Geometry: final body of the model. Coordinates: model frame, mm. A direction names the side the tool comes from. Round coordinates to 2 decimals unless told otherwise and drop trailing zeros. Loops run counter-clockwise (first coordinate to the right, second up) from the corner with the lowest first, then second, coordinate; pieces in that order, holes last. Notation, with made-up numbers: M 20,40.25 L 55,40.25 A25 cw 55,56.25 Z; hole C -37,5 d11. An arc over 180 degrees is marked long. Answer as a JSON object with one key per item and string values.
from build123d import *

# Parameters (mm, degrees)
F1_DEPTH = 1
F2_DEPTH = 11
F3_DEPTH = 10


with BuildPart() as f1:
    # F0 (on Top) → F1 (new body)
    with BuildSketch(Plane.XY):
        with BuildLine():
            ThreePointArc((12.3109959605, -2.4885695612), (12.4975939537, -1.250498048), (12.56, 0))
            ThreePointArc((12.56, 0), (12.499849565, 1.227746249), (12.3199743866, 2.4437330282))
            ThreePointArc((12.3199743866, 2.4437330282), (8.8241351782, 8.9380220607), (2.2855528975, 12.3502974844))
            ThreePointArc((2.2855528975, 12.3502974844), (0.0100228873, 12.5599960009), (-2.2658389037, 12.3539294988))
            ThreePointArc((-2.2658389037, 12.3539294988), (-8.8620220769, 8.9004586797), (-12.3440076572, 2.3192832854))
            ThreePointArc((-12.3440076572, 2.3192832854), (-12.559977123, 0.023972266), (-12.3527709674, -2.2721464362))
            ThreePointArc((-12.3527709674, -2.2721464362), (-8.8868925427, -8.8756262277), (-2.2878147001, -12.3498786997))
            ThreePointArc((-2.2878147001, -12.3498786997), (0.0002376292, -12.5599999978), (2.2882820061, -12.3497921222))
            ThreePointArc((2.2882820061, -12.3497921222), (8.8088397015, -8.9530968449), (12.3109959605, -2.4885695612))
        make_face()
        with BuildLine():
            ThreePointArc((12.3199743866, 2.4437330282), (12.499849565, 1.227746249), (12.56, 0))
            ThreePointArc((12.56, 0), (12.4975939537, -1.250498048), (12.3109959605, -2.4885695612))
            Line((12.3109959605, -2.4885695612), (13.1075011071, -2.5855424186))
            Line((13.1075011071, -2.5855424186), (14.1026028651, -2.7066940036))
            ThreePointArc((14.1026028651, -2.7066940036), (14.2955058872, -1.3594526209), (14.36, 0))
            ThreePointArc((14.36, 0), (14.2978344087, 1.334740133), (14.1118758743, 2.657923872))
            Line((14.1118758743, 2.657923872), (13.1166017889, 2.5389560617))
            Line((13.1166017889, 2.5389560617), (12.3199743866, 2.4437330282))
        make_face()
        with BuildLine():
            ThreePointArc((2.2855528975, 12.3502974844), (8.8241351782, 8.9380220607), (12.3199743866, 2.4437330282))
            Line((12.3199743866, 2.4437330282), (13.1166017889, 2.5389560617))
            Line((13.1166017889, 2.5389560617), (14.1118758743, 2.657923872))
            ThreePointArc((14.1118758743, 2.657923872), (10.136505033, 10.1715714477), (2.6091735777, 14.1209706905))
            Line((2.6091735777, 14.1209706905), (2.4293843449, 13.1372635399))
            Line((2.4293843449, 13.1372635399), (2.2855528975, 12.3502974844))
        make_face()
        with BuildLine():
            Line((13.1075011071, -2.5855424186), (12.3109959605, -2.4885695612))
            ThreePointArc((12.3109959605, -2.4885695612), (8.8088397015, -8.9530968449), (2.2882820061, -12.3497921222))
            Line((2.2882820061, -12.3497921222), (2.4340324524, -13.1364030853))
            Line((2.4340324524, -13.1364030853), (2.6162205102, -14.1196667893))
            ThreePointArc((2.6162205102, -14.1196667893), (10.1214500303, -10.1865523748), (14.1026028651, -2.7066940036))
            Line((14.1026028651, -2.7066940036), (13.1075011071, -2.5855424186))
        make_face()
        with BuildLine():
            ThreePointArc((-2.2658389037, 12.3539294988), (0.0100228873, 12.5599960009), (2.2855528975, 12.3502974844))
            Line((2.2855528975, 12.3502974844), (2.4293843449, 13.1372635399))
            Line((2.4293843449, 13.1372635399), (2.6091735777, 14.1209706905))
            ThreePointArc((2.6091735777, 14.1209706905), (-0.0077642493, 14.359997901), (-2.624442069, 14.118140948))
            Line((-2.624442069, 14.118140948), (-2.4252208949, 13.1380372835))
            Line((-2.4252208949, 13.1380372835), (-2.2658389037, 12.3539294988))
        make_face()
        with BuildLine():
            Line((2.4340324524, -13.1364030853), (2.2882820061, -12.3497921222))
            ThreePointArc((2.2882820061, -12.3497921222), (0.0002376292, -12.5599999978), (-2.2878147001, -12.3498786997))
            Line((-2.2878147001, -12.3498786997), (-2.431047805, -13.136955882))
            Line((-2.431047805, -13.136955882), (-2.6100890312, -14.1208015087))
            ThreePointArc((-2.6100890312, -14.1208015087), (0.0031177966, -14.3599996615), (2.6162205102, -14.1196667893))
            Line((2.6162205102, -14.1196667893), (2.4340324524, -13.1364030853))
        make_face()
        with BuildLine():
            ThreePointArc((-12.3440076572, 2.3192832854), (-8.8620220769, 8.9004586797), (-2.2658389037, 12.3539294988))
            Line((-2.2658389037, 12.3539294988), (-2.4252208949, 13.1380372835))
            Line((-2.4252208949, 13.1380372835), (-2.624442069, 14.118140948))
            ThreePointArc((-2.624442069, 14.118140948), (-10.146271601, 10.1618291955), (-14.1141033231, 2.6460701775))
            Line((-14.1141033231, 2.6460701775), (-13.1307172202, 2.4645219739))
            Line((-13.1307172202, 2.4645219739), (-12.3440076572, 2.3192832854))
        make_face()
        with BuildLine():
            Line((-2.431047805, -13.136955882), (-2.2878147001, -12.3498786997))
            ThreePointArc((-2.2878147001, -12.3498786997), (-8.8868925427, -8.8756262277), (-12.3527709674, -2.2721464362))
            Line((-12.3527709674, -2.2721464362), (-14.1224720777, -2.601034874))
            ThreePointArc((-14.1224720777, -2.601034874), (-10.1573080166, -10.1507976955), (-2.6100890312, -14.1208015087))
            Line((-2.6100890312, -14.1208015087), (-2.431047805, -13.136955882))
        make_face()
        with BuildLine():
            ThreePointArc((-12.3527709674, -2.2721464362), (-12.559977123, 0.023972266), (-12.3440076572, 2.3192832854))
            Line((-12.3440076572, 2.3192832854), (-13.1307172202, 2.4645219739))
            Line((-13.1307172202, 2.4645219739), (-14.1141033231, 2.6460701775))
            ThreePointArc((-14.1141033231, 2.6460701775), (-14.3599817356, 0.0229031363), (-14.1224720777, -2.601034874))
            Line((-14.1224720777, -2.601034874), (-12.3527709674, -2.2721464362))
        make_face()
    extrude(amount=F1_DEPTH)

    # F0 (on Top) → F2 (join)
    with BuildSketch(Plane.XY):
        with BuildLine():
            ThreePointArc((2.2855528975, 12.3502974844), (8.8241351782, 8.9380220607), (12.3199743866, 2.4437330282))
            Line((12.3199743866, 2.4437330282), (13.1166017889, 2.5389560617))
            Line((13.1166017889, 2.5389560617), (14.1118758743, 2.657923872))
            ThreePointArc((14.1118758743, 2.657923872), (10.136505033, 10.1715714477), (2.6091735777, 14.1209706905))
            Line((2.6091735777, 14.1209706905), (2.4293843449, 13.1372635399))
            Line((2.4293843449, 13.1372635399), (2.2855528975, 12.3502974844))
        make_face()
        with BuildLine():
            Line((13.1075011071, -2.5855424186), (12.3109959605, -2.4885695612))
            ThreePointArc((12.3109959605, -2.4885695612), (8.8088397015, -8.9530968449), (2.2882820061, -12.3497921222))
            Line((2.2882820061, -12.3497921222), (2.4340324524, -13.1364030853))
            Line((2.4340324524, -13.1364030853), (2.6162205102, -14.1196667893))
            ThreePointArc((2.6162205102, -14.1196667893), (10.1214500303, -10.1865523748), (14.1026028651, -2.7066940036))
            Line((14.1026028651, -2.7066940036), (13.1075011071, -2.5855424186))
        make_face()
        with BuildLine():
            ThreePointArc((-12.3440076572, 2.3192832854), (-8.8620220769, 8.9004586797), (-2.2658389037, 12.3539294988))
            Line((-2.2658389037, 12.3539294988), (-2.4252208949, 13.1380372835))
            Line((-2.4252208949, 13.1380372835), (-2.624442069, 14.118140948))
            ThreePointArc((-2.624442069, 14.118140948), (-10.146271601, 10.1618291955), (-14.1141033231, 2.6460701775))
            Line((-14.1141033231, 2.6460701775), (-13.1307172202, 2.4645219739))
            Line((-13.1307172202, 2.4645219739), (-12.3440076572, 2.3192832854))
        make_face()
        with BuildLine():
            ThreePointArc((2.6091735777, 14.1209706905), (10.136505033, 10.1715714477), (14.1118758743, 2.657923872))
            Line((14.1118758743, 2.657923872), (14.7487280331, 2.7340485374))
            ThreePointArc((14.7487280331, 2.7340485374), (10.6030739469, 10.6101283158), (2.7242386681, 14.7505431656))
            Line((2.7242386681, 14.7505431656), (2.6091735777, 14.1209706905))
        make_face()
        with BuildLine():
            Line((-2.431047805, -13.136955882), (-2.2878147001, -12.3498786997))
            ThreePointArc((-2.2878147001, -12.3498786997), (-8.8868925427, -8.8756262277), (-12.3527709674, -2.2721464362))
            Line((-12.3527709674, -2.2721464362), (-14.1224720777, -2.601034874))
            ThreePointArc((-14.1224720777, -2.601034874), (-10.1573080166, -10.1507976955), (-2.6100890312, -14.1208015087))
            Line((-2.6100890312, -14.1208015087), (-2.431047805, -13.136955882))
        make_face()
        with BuildLine():
            Line((14.7393400257, -2.7842154385), (14.1026028651, -2.7066940036))
            ThreePointArc((14.1026028651, -2.7066940036), (10.1214500303, -10.1865523748), (2.6162205102, -14.1196667893))
            Line((2.6162205102, -14.1196667893), (2.7328208672, -14.7489555599))
            ThreePointArc((2.7328208672, -14.7489555599), (10.5880995986, -10.6250716181), (14.7393400257, -2.7842154385))
        make_face()
        with BuildLine():
            ThreePointArc((-14.1141033231, 2.6460701775), (-10.146271601, 10.1618291955), (-2.624442069, 14.118140948))
            Line((-2.624442069, 14.118140948), (-2.7519420936, 14.7453997814))
            ThreePointArc((-2.7519420936, 14.7453997814), (-10.6028895523, 10.6103125845), (-14.7434702232, 2.7622609899))
            Line((-14.7434702232, 2.7622609899), (-14.1141033231, 2.6460701775))
        make_face()
        with BuildLine():
            ThreePointArc((-2.6100890312, -14.1208015087), (-10.1573080166, -10.1507976955), (-14.1224720777, -2.601034874))
            Line((-14.1224720777, -2.601034874), (-14.7516989871, -2.717972957))
            ThreePointArc((-14.7516989871, -2.717972957), (-10.6090110951, -10.6041917931), (-2.7246753784, -14.750462504))
            Line((-2.7246753784, -14.750462504), (-2.6100890312, -14.1208015087))
        make_face()
    extrude(amount=-F2_DEPTH)

    # F0 (on Top) → F3 (cut)
    with BuildSketch(Plane.XY):
        with BuildLine():
            ThreePointArc((-14.1141033231, 2.6460701775), (-10.146271601, 10.1618291955), (-2.624442069, 14.118140948))
            Line((-2.624442069, 14.118140948), (-2.7519420936, 14.7453997814))
            ThreePointArc((-2.7519420936, 14.7453997814), (-10.6028895523, 10.6103125845), (-14.7434702232, 2.7622609899))
            Line((-14.7434702232, 2.7622609899), (-14.1141033231, 2.6460701775))
        make_face()
        with BuildLine():
            ThreePointArc((2.6091735777, 14.1209706905), (10.136505033, 10.1715714477), (14.1118758743, 2.657923872))
            Line((14.1118758743, 2.657923872), (14.7487280331, 2.7340485374))
            ThreePointArc((14.7487280331, 2.7340485374), (10.6030739469, 10.6101283158), (2.7242386681, 14.7505431656))
            Line((2.7242386681, 14.7505431656), (2.6091735777, 14.1209706905))
        make_face()
        with BuildLine():
            Line((14.7393400257, -2.7842154385), (14.1026028651, -2.7066940036))
            ThreePointArc((14.1026028651, -2.7066940036), (10.1214500303, -10.1865523748), (2.6162205102, -14.1196667893))
            Line((2.6162205102, -14.1196667893), (2.7328208672, -14.7489555599))
            ThreePointArc((2.7328208672, -14.7489555599), (10.5880995986, -10.6250716181), (14.7393400257, -2.7842154385))
        make_face()
        with BuildLine():
            ThreePointArc((-2.6100890312, -14.1208015087), (-10.1573080166, -10.1507976955), (-14.1224720777, -2.601034874))
            Line((-14.1224720777, -2.601034874), (-14.7516989871, -2.717972957))
            ThreePointArc((-14.7516989871, -2.717972957), (-10.6090110951, -10.6041917931), (-2.7246753784, -14.750462504))
            Line((-2.7246753784, -14.750462504), (-2.6100890312, -14.1208015087))
        make_face()
    extrude(amount=-F3_DEPTH, mode=Mode.SUBTRACT)


solid = f1.part
1) Pin query (flat end, axial travel): P1, Ø3, axis at y = 9.5, z = -6, coming from the +X side; P2, Ø4, axis at x = -11.5, z = -8.5, coming from the -Y side; P3, Ø8.5, axis at x = 0.5, y = -2, coming from the -Z side. Return the tip coordinate at first contact, or that it passes through.
Results:
{"P1": "x = 11.93", "P2": "y = -11.02", "P3": "z = 0"}
2) Section query C-C (y = -9.75). Return the cut outline in (x, z), and give its area (3 significant figures).
Results:
{"outline": "M -11.4,-11 L -7.92,-11 L -7.92,0 L 7.92,0 L 7.92,-11 L 11.4,-11 L 11.4,-10 L 10.54,-10 L 10.54,1 L -10.54,1 L -10.54,-10 L -11.4,-10 Z", "area": "80.5 mm2"}
3) Reachability of faces 1 (the flat face through (10, 10.52, -10)), 2 (the flat face through (10.4, -10.5, -10)), 3 (the flat face through (-10.5, -10.4, -10)), 4 (the cylindrical face through (-8.81, -8.95, -5.42)), 5 (the flat face through (-10.1, 10.5, -10)) from +Z, -Z, +X, -X, +Y, -Y: full face, straight path, thin tool, end or side. Return the list, or none.
Results:
{"face 1": "+Z, +X, +Y", "face 2": "+Z, +X, -Y", "face 3": "+Z, -X, -Y", "face 4": "-Z", "face 5": "+Z, -X, +Y"}
4) Ray query, line 1 (Z direction, x = 8, y = 5.25); line 2 (Y direction, x = -2.75, z = -5); line 3 (Y direction, x = -10.25, z = -4.25). Return the intervals inside material, ascending.
Results:
{"line 1": "0 to 1", "line 2": "-14.09 to -12.26, 12.26 to 14.09", "line 3": "-10.06 to -7.26, 7.26 to 10.06"}
5) Section query B-B (x = 10.25). Return the cut outline in (y, z), and give its area (3 significant figures).
Results:
{"outline": "M -10.95,-11 L -7.26,-11 L -7.26,0 L 7.26,0 L 7.26,-11 L 10.95,-11 L 10.95,-10 L 10.06,-10 L 10.06,1 L -10.06,1 L -10.06,-10 L -10.95,-10 Z", "area": "83.5 mm2"}
6) Pull-direction query (Y, two-part tool) for faces 6 (the cylindrical face through (10.69, 10.52, -10.49)), 7 (the cylindrical face through (8.88, -8.88, -5.42)), 8 (the flat face through (9, 9, -11)); classes: +Y half, -Y half, draft (parallel to the pull), parting line (faces both ways), or undercut.
Results:
{"face 6": "+Y half", "face 7": "undercut", "face 8": "draft"}
7) Section query A-A (z = -2.5). Return the cut outline in (x, y), and give its area (3 significant figures).
Results:
{"outline": "M -14.12,-2.6 A14.36 ccw -2.61,-14.12 L -2.29,-12.35 A12.56 cw -12.35,-2.27 Z; M -14.11,2.65 L -12.34,2.32 A12.56 cw -2.27,12.35 L -2.62,14.12 A14.36 ccw Z; M 2.29,-12.35 L 2.62,-14.12 A14.36 ccw 14.1,-2.71 L 12.31,-2.49 A12.56 cw Z; M 2.29,12.35 A12.56 cw 12.32,2.44 L 14.11,2.66 A14.36 ccw 2.61,14.12 Z", "area": "116 mm2"}
